Read the model definition and answer for the solid it produces. Units are mm, in the model's axes. A direction names the side the tool comes from. Coordinates: 2 decimals unless noted, no trailing zeros. Loops run counter-clockwise (first coordinate to the right, second up) from the corner with the lowest first, then second, coordinate; pieces in that order, holes last. Notation, with made-up numbers: (76.25, -35.75) -> (81.25, -35.75) arc R25 ccw to (81.25, -12.75) -> close; hole circle Ø2 at (-26.75, 7). An arc over 180 degrees is marked (long way). Answer as a JSON object with one key per item and string values. Group by question number.
1) Which of the six approach directions +Z, -Z, +X, -X, +Y, -Y give full straight-line access (tool end or side, diameter ignored) to faces 1 (the face through (-61.99, 1043.89, -13.77)), 2 (the face through (-75.59, 1.23, -16.79))?
2) Consider probe 1 along Y at (x, z) = (-46, 54.5); probe 2 along Z at (x, y) = (-4, 1167); probe 3 along X at (y, z) = (188, -1). Determine where each line is inside the solid, lowest interval first. Write a range as [from, to].
3) Flat-ended cylindrical pins translate along their axes: P1, Ø1, axis at x = -69.5, y = 346.5, coming from the -Z side; P2, Ø8, axis at x = -65.5, y = 557.5, coming from the +Z side; P3, Ø8, axis at y = 950.5, z = -7.5, coming from the -X side; P4, Ø3, axis at x = 3.5, z = 60, coming from the -Y side. Find the tip coordinate at first contact, or state that the pin passes through.
4) Section A-A, the plane x = 0 is taken. Give the vertices of the cut face in (y, z).
5) Section D-D, the plane y = 975.5 is taken. Give the vertices of the cut face in (x, z).
6) Section C-C, the plane y = 289 is taken. Give the vertices of the cut face in (x, z).
7) Section B-B, the plane z = 0 is taken. Give the vertices of the cut face in (x, y).
from build123d import *

# Parameters (mm, degrees)
SKETCH1_R           = 101.6
BOSS_EXTRUDE1_DEPTH = 1219.2
SKETCH2_OUTSIDE_W   = 455.722
SKETCH2_OUTSIDE_H   = 455.722
SKETCH2_OUTSIDE_R   = 63.5
CUT_EXTRUDE1_DEPTH  = 355.6
CHAMFER1_SIZE       = 25.4


with BuildPart() as part:
    # Sketch1 → Boss-Extrude1 (new body)
    with BuildSketch(Plane(origin=(0, 0, 0), x_dir=(1, 0, 0), z_dir=(0, 1, 0))):
        with Locations(Location((0, 0, 0), (0, 0, 270))):  # turned: the seam where the file's is
            Circle(SKETCH1_R)
    extrude(amount=BOSS_EXTRUDE1_DEPTH)

    # Sketch2 outside → Cut-Extrude1 (cut)
    with BuildSketch(Plane(origin=(0, 1219.2, 0), x_dir=(1, 0, 0), z_dir=(0, 1, 0))):
        Rectangle(SKETCH2_OUTSIDE_W, SKETCH2_OUTSIDE_H)
        with Locations(Location((0, 0, 0), (0, 0, 270))):  # turned: the seam where the file's is
            Circle(SKETCH2_OUTSIDE_R, mode=Mode.SUBTRACT)
    extrude(amount=-CUT_EXTRUDE1_DEPTH, mode=Mode.SUBTRACT)

    # Chamfer1
    chamfer1_edges = [part.edges().sort_by_distance(p)[0] for p in [
        (0, 0, -101.6),
    ]]
    chamfer(chamfer1_edges, length=CHAMFER1_SIZE)


solid = part.part
Determined:
{
 "1": {"face 1": "+Y", "face 2": "-Y"},
 "2": {"probe 1": "[0, 863.6]", "probe 2": "[-63.37, 63.37]", "probe 3": "[-101.6, 101.6]"},
 "3": {"P1": "z = -74.58", "P2": "z = 80.87", "P3": "x = -63.4", "P4": "y = 0"},
 "4": {"outline": "(0, -76.2) -> (25.4, -101.6) -> (863.6, -101.6) -> (863.6, -63.5) -> (1219.2, -63.5) -> (1219.2, 63.5) -> (863.6, 63.5) -> (863.6, 101.6) -> (25.4, 101.6) -> (0, 76.2) -> close"},
 "5": {"outline": "circle Ø127 at (0, 0)"},
 "6": {"outline": "circle Ø203.2 at (0, 0)"},
 "7": {"outline": "(-101.6, 25.4) -> (-76.2, 0) -> (76.2, 0) -> (101.6, 25.4) -> (101.6, 863.6) -> (63.5, 863.6) -> (63.5, 1219.2) -> (-63.5, 1219.2) -> (-63.5, 863.6) -> (-101.6, 863.6) -> close"}
}
